Build history of the part. All positions in model axes, mm. A direction names the side the tool comes from. Coordinates: 2 decimals unless noted, no trailing zeros. Order: outer loops, then holes, each group sorted by start corner. A loop starts at its lowest first (then second) coordinate and runs counter-clockwise, first axis right, second up. Notation, with made-up numbers: (39, 73.25) - (55, 73.25) arc R24 cw to (55, 106.25) - close; hole circle Ø9 at (-40, 46.5). An arc over 180 degrees is marked (long way). Return JSON: item names as keys, results as strings.
Autodesk Inventor part; units mm, degrees
ref_plane "YZ Plane" through (0, 0, 0) normal (1, 0, 0) x (0, 1, 0)
ref_plane "XZ Plane" through (0, 0, 0) normal (0, 1, 0) x (-1, 0, 0)
ref_plane "XY Plane" through (0, 0, 0) normal (0, 0, 1) x (1, 0, 0)
sketch "Sketch1" plane through (0, 0, 0) normal (0, 0, 1) x (1, 0, 0)
  line L0 (31.1987, 43.9856) -> (69.7487, 43.9856)
  line L1 (69.7487, 43.9856) -> (69.7487, -56.0144)
  line L2 (69.7487, -56.0144) -> (31.1987, -56.0144)
  line L3 (31.1987, -56.0144) -> (31.1987, 43.9856)
  point P0 (0, 0)
  dimension "d0" = 100
  dimension "d1" = 38.55
extrude "Plate1" add sketch "Sketch1" along normal blind 0.5
sketch "Sketch2" plane through (31.6987, -56.0144, 0) normal (-1, 0, 0) x (0, -1, 0)
  line L0 (-100, 0) -> (0, 0)
  line L1 (0, 0) -> (0, 22)
  line L2 (0, 22) -> (-100, 22)
  line L3 (-100, 22) -> (-100, 0)
edge flange "Flange1" height 22 angle 90 thickness 0.5 bend radius 0.5 thickness toward (-1, 0, 0) relief tear relief width 0.5 relief depth 0.25 edges at (31.1987, -6.0144, 0.5) wall of the first edge with corners at (31.6987, 43.9856, 0) (31.6987, -56.0144, 0) (31.6987, -56.0144, 22) (31.6987, 43.9856, 22)
bend "Bend1"
corner "Corner1"
sketch "Sketch3" plane through (31.6987, 43.9856, 21.5) normal (0, 0, 1) x (1, 0, 0)
  line L0 (0, -100) -> (0, 0)
  line L1 (0, 0) -> (-100, 0)
  line L2 (-100, 0) -> (-100, -100)
  line L3 (-100, -100) -> (0, -100)
edge flange "Flange2" height 100 angle 90 thickness 0.5 bend radius 0.5 thickness toward (0, 0, 1) relief tear relief width 0.5 relief depth 0.25 edges at (31.1987, -6.0144, 22) wall of the first edge with corners at (31.6987, -56.0144, 21.5) (31.6987, 43.9856, 21.5) (-68.3013, 43.9856, 21.5) (-68.3013, -56.0144, 21.5)
bend "Bend2"
corner "Corner2"
sketch "Sketch4" plane through (0, 0, 0.5) normal (0, 0, 1) x (1, 0, 0)
  line L0 (48.2487, 25.2184) -> (48.2487, -36.8148) construction
  line L1 (32.1987, 43.9856) -> (69.7487, 43.9856)
  line L2 (69.7487, -56.0144) -> (32.1987, -56.0144)
  line L3 (69.7487, 43.9856) -> (69.7487, -56.0144)
  point P0 (0, 0)
  point P1 (48.2487, 24.9856)
  point P2 (48.2487, -37.0144)
  dimension "d23" = 19
  dimension "d24" = 62
  dimension "d25" = 19
  dimension "d26" = 21.5
hole "Hole1" at (48.2487, 24.9856, 0.5) at (48.2487, -37.0144, 0.5) direction (0, 0, -1) diameter 5.1 end through all
sketch "Sketch5" plane through (-68.3013, -56.0144, 22) normal (0, 0, 1) x (1, 0, 0)
  line L0 (84, 64.1) -> (84, 35.9) construction
  line L1 (0, 100) -> (99, 100)
  line L2 (99, 0) -> (0, 0)
  line L3 (99, 0) -> (99, 100)
  point P0 (68.3013, 56.0144)
  dimension "d34" = 28.2
  dimension "d35" = 35.9
  dimension "d36" = 35.9
  dimension "d37" = 15
hole "Hole2" at (15.6987, 8.0856, 22) at (15.6987, -20.1144, 22) direction (0, 0, -1) diameter 4.1 end through all
sketch "Sketch6" plane through (-68.3013, -56.0144, 22) normal (0, 0, 1) x (1, 0, 0)
  line L0 (5, 95) -> (5, 75) construction
  line L1 (0, 100) -> (99, 100)
  line L2 (0, 0) -> (0, 100)
  point P0 (68.3013, 56.0144)
  dimension "d45" = 20
  dimension "d46" = 5
  dimension "d47" = 5
hole "Hole3" at (-63.3013, 38.9856, 22) at (-63.3013, 18.9856, 22) direction (0, 0, -1) diameter 5.1 end through all
equation "\"d32\" = Thickness"
equation "\"d35\" = d36"
equation "\"d2\" = Thickness"
equation "\"d3\" = BendReliefWidth"
equation "\"d4\" = BendReliefDepth"
equation "\"d5\" = MinimumRemnant"
equation "\"d6\" = TransitionRadius"
equation "\"d9\" = BendRadius"
equation "\"d10\" = CornerReliefSize"
equation "\"d11\" = GapSize"
equation "\"d12\" = JacobiRadiusSize"
equation "\"d13\" = BendReliefWidth"
equation "\"d14\" = BendReliefDepth"
equation "\"d15\" = MinimumRemnant"
equation "\"d16\" = TransitionRadius"
equation "\"d19\" = BendRadius"
equation "\"d20\" = CornerReliefSize"
equation "\"d21\" = GapSize"
equation "\"d22\" = JacobiRadiusSize"
equation "\"BendRadius\" = Thickness"
equation "\"BendReliefWidth\" = Thickness"
equation "\"BendReliefDepth\" = 0.5 * Thickness"
equation "\"CornerReliefSize\" = 4 * Thickness"
equation "\"MinimumRemnant\" = 2 * Thickness"
equation "\"TransitionRadius\" = BendRadius"
equation "\"JacobiRadiusSize\" = BendRadius"
equation "\"GapSize\" = Thickness"
properties part number "Placa Montaje"
1. Cut at A-A on y = -14.5. Give the cut face in (x, z).
Check values:
{"outline": "(-68.3, 21.5) - (30.7, 21.5) arc R0.5 cw to (31.2, 21) - (31.2, 1) arc R1 ccw to (32.2, 0) - (69.75, 0) - (69.75, 0.5) - (32.2, 0.5) arc R0.5 cw to (31.7, 1) - (31.7, 21) arc R1 ccw to (30.7, 22) - (-68.3, 22) - close"}
2. Probe L1, parallel to X at y = 38.5, z = 2.75; L2, parallel to Z at x = 8, y = -40; L3, parallel to Z at x = 38, y = -7.5. List the from-to ranges inside material, lowest first.
Check values:
{"L1": "31.2 to 31.7", "L2": "21.5 to 22", "L3": "0 to 0.5"}
3. Cut at C-C on x = 20.5. Give the cut face in (y, z).
Check values:
{"outline": "(-56.01, 21.5) - (43.99, 21.5) - (43.99, 22) - (-56.01, 22) - close"}
4. Tool access for faces 3 (the flat face through (51, -5, 0.5)), 4 (the flat face through (-18, -5, 21.5)), 5 (the cylindrical face through (-65.83, 19.32, 21.75)): list every direction of +Z, -Z, +X, -X, +Y, -Y with a clear straight run to the whole face (end or side of a thin tool).
Check values:
{"face 3": "+Z, +X, +Y, -Y", "face 4": "-Z, -X, +Y, -Y", "face 5": "+Z, -Z"}
5. Cut at B-B on z = 3. Give the cut face in (x, y), plus the area to 3 significant figures.
Check values:
{"outline": "(31.2, -56.01) - (31.7, -56.01) - (31.7, 43.99) - (31.2, 43.99) - close", "area": "50.0 mm²"}
6. Mould opens along Y. For faces 1 (the cylindrical face through (46.53, -35.13, 0.25)), 2 (the flat face through (-19, -5, 22)) say: pulls with the +Y half, pulls with the -Y half, needs draft (parallel to the pull), parting line crosses it, or undercut.
Check values:
{"face 1": "undercut", "face 2": "needs draft"}
7. Drop flat-ended pins along their axis: pin 1 (19 mm diameter, centred on x = 48.5, y = 10.5, fed in from +Z); pin 2 (2 mm diameter, centred on x = 21, y = -10.5, fed in from -Z); pin 3 (8 mm diameter, centred on y = 33, z = 9, fed in from -X). Give the stop position or say it passes through.
Check values:
{"pin 1": "z = 0.5", "pin 2": "z = 21.5", "pin 3": "x = 31.2"}
